Verification items for the finished model (mm, model axes). Round coordinates to 2 decimals unless told otherwise and drop trailing zeros. Write each loop counter-clockwise with the first axis right and the second up, starting at its lowest first coordinate (ties: lowest second). Pieces come first, ordered by that corner, then holes. Notation, with made-up numbers: M -36,19.5 L -31,19.5 A18 ccw -31,43.5 Z; hole C 81,-36 d2. An arc over 180 degrees is marked long. Write each question's results on one line, items separated by ' | '.
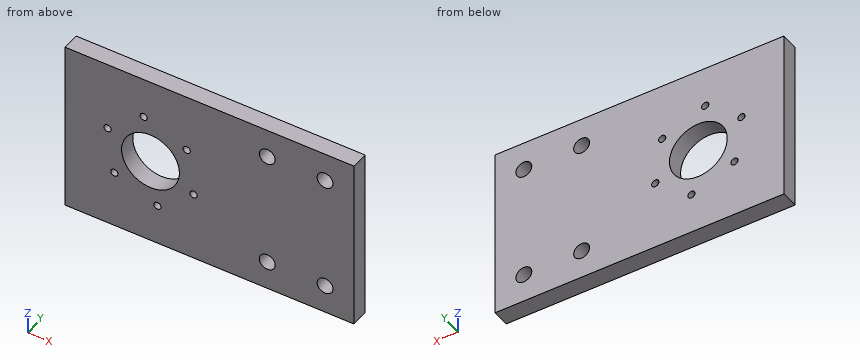
from build123d import *

# Parameters (mm, degrees)
SKETCH1_W           = 100
SKETCH1_H           = 60
BOSS_EXTRUDE1_DEPTH = 6
SKETCH2_R           = 10
SKETCH2_R_2         = 2.75
CUT_EXTRUDE1_DEPTH  = 6
SKETCH3_R           = 1.25
CUT_EXTRUDE2_DEPTH  = 7


with BuildPart() as part:
    # Sketch1 → Boss-Extrude1 (new body)
    with BuildSketch(Plane(origin=(0, 0, 0), x_dir=(1, 0, 0), z_dir=(0, 1, 0))):
        with Locations((50, 30)):
            Rectangle(SKETCH1_W, SKETCH1_H)
    extrude(amount=BOSS_EXTRUDE1_DEPTH)

    # Sketch2 → Cut-Extrude1 (cut)
    with BuildSketch(Plane(origin=(0, 6, 0), x_dir=(1, 0, 0), z_dir=(0, 1, 0))):
        with Locations((29.615341175, 30)):
            Circle(SKETCH2_R)
        with Locations((70, 50)):
            Circle(SKETCH2_R_2)
        with Locations((90, 50)):
            Circle(SKETCH2_R_2)
        with Locations((70, 10)):
            Circle(SKETCH2_R_2)
        with Locations((90, 10)):
            Circle(SKETCH2_R_2)
    extrude(amount=-CUT_EXTRUDE1_DEPTH, mode=Mode.SUBTRACT)

    # Sketch3 → Cut-Extrude2 (cut, through all)
    with BuildSketch(Plane(origin=(0, 6, 0), x_dir=(1, 0, 0), z_dir=(0, 1, 0))):
        with Locations((31.998383025, 45.821539481)):
            Circle(SKETCH3_R)
        with Locations((44.508717217, 35.846994961)):
            Circle(SKETCH3_R)
        with Locations((42.125675368, 20.02545548)):
            Circle(SKETCH3_R)
        with Locations((27.232299326, 14.178460519)):
            Circle(SKETCH3_R)
        with Locations((14.721965133, 24.153005039)):
            Circle(SKETCH3_R)
        with Locations((17.105006983, 39.97454452)):
            Circle(SKETCH3_R)
    extrude(amount=-CUT_EXTRUDE2_DEPTH, mode=Mode.SUBTRACT)


solid = part.part
1) Material ranges on line 1 (X direction, y = 1.4, z = -50); line 2 (Z direction, x = 70, y = 2.6); line 3 (Z direction, x = 17, y = 1.55), recorded low to high. Write a range as [from, to].
Calculated:
line 1: x = [0, 67.25], [72.75, 87.25], [92.75, 100] | line 2: z = [-60, -52.75], [-47.25, -12.75], [-7.25, 0] | line 3: z = [-60, -41.22], [-38.73, 0]
2) Sectioned sample at A-A, the plane z = -10. Record the cut outline in (x, y).
Calculated:
outline: M 0,0 L 67.25,0 L 67.25,6 L 0,6 Z; M 72.75,0 L 87.25,0 L 87.25,6 L 72.75,6 Z; M 92.75,0 L 100,0 L 100,6 L 92.75,6 Z
3) Sectioned sample at B-B, the plane x = 70. Record the cut outline in (y, z), and give its area (3 significant figures).
Calculated:
outline: M 0,-60 L 6,-60 L 6,-52.75 L 0,-52.75 Z; M 0,-47.25 L 6,-47.25 L 6,-12.75 L 0,-12.75 Z; M 0,-7.25 L 6,-7.25 L 6,0 L 0,0 Z | area: 294 mm²
4) Sectioned sample at C-C, the plane y = 4.65. Count the separate pieces of the cut face and the enclosed holes in it, and give its area (3 significant figures).
Calculated:
separate pieces: 1 | enclosed holes: 11 | area: 5,560 mm²
